from build123d import *

# Parameters (mm, degrees)
SKETCH1_R           = 8.89
SKETCH1_R_2         = 6.35
BOSS_EXTRUDE1_DEPTH = 13.462
SKETCH3_R           = 8.89
SKETCH3_R_2         = 6.35
SKETCH5_R           = 8.89
SKETCH5_R_2         = 6.349329507
BOSS_EXTRUDE2_DEPTH = 13.462


with BuildPart() as part:
    # Sketch1 → Boss-Extrude1 (new body)
    with BuildSketch(Plane(origin=(0, 0, 0), x_dir=(1, 0, 0), z_dir=(0, 1, 0))):
        with Locations(Location((0, 0, 0), (0, 0, 270))):
            Circle(SKETCH1_R)
        with Locations(Location((0, 0, 0), (0, 0, 270))):
            Circle(SKETCH1_R_2, mode=Mode.SUBTRACT)
    extrude(amount=BOSS_EXTRUDE1_DEPTH)

    # Sweep1: sweep along a path in Sketch2
    with BuildLine(Plane(origin=(0, 0, 0), x_dir=(0, 0, -1), z_dir=(1, 0, 0))) as sweep1_path:
        ThreePointArc((0, 0), (-3.719743879, -8.980256121), (-12.7, -12.7))
    # Sketch3 → Sweep1 (sweep)
    with BuildSketch(Plane.XZ):
        Circle(SKETCH3_R)
        Circle(SKETCH3_R_2, mode=Mode.SUBTRACT)
    sweep(path=sweep1_path.line)

    # Sketch5 → Boss-Extrude2 (add)
    with BuildSketch(Plane.XY.offset(12.7)):
        with Locations(Location((0, -12.7, 0), (0, 0, 270))):
            Circle(SKETCH5_R)
        with Locations(Location((0, -12.7, 0), (0, 0, 270))):
            Circle(SKETCH5_R_2, mode=Mode.SUBTRACT)
    extrude(amount=BOSS_EXTRUDE2_DEPTH)


solid = part.part
Geometry: final body of the model. Coordinates: model frame, mm. A direction names the side the tool comes from. Give positions to 0.01 mm unless a question says otherwise; leave off trailing zeros. Loops run counter-clockwise (first coordinate to the right, second up) from the corner with the lowest first, then second, coordinate; pieces in that order, holes last. Notation, with made-up numbers: (0.5, -6) - (16.5, -6) arc R10 ccw to (16.5, 12) - close; hole circle Ø2 at (10, 76). An arc over 180 degrees is marked (long way). One line per question, with ' | ' between items. Start each with the question number.
(1) Section query B-B on y = 4. Return loops of the section in (x, z).
(2) Ray query, line 1 (Y direction, x = 0, z = 23); line 2 (X direction, y = -12.7, z = 19.25); line 3 (Z direction, x = 2, y = 7). Return the intervals inside material, ascending. Write a range as from..to.
(3) Section query D-D on x = 7. Return loops of the section in (y, z).
(4) Reachability of faces 4 (the cylindrical face through (-8.68, 6.64, -1.93)), 5 (the flat face through (-6, 13.462, 4)), 6 (the cylindrical face through (-3.86, -7.66, 19.34)) from +Z, -Z, +X, -X, +Y, -Y: full face, straight path, thin tool, end or side. Return the list, or none.
(5) Contact query for flat-ended pins moving along their axis: pin 1 (1 mm diameter, centred on x = -2, y = -17, fed in from -Z); pin 2 (1.5 mm diameter, centred on x = -2.5, y = -12.5, fed in from -Z); pin 3 (2 mm diameter, centred on x = 0.5, y = -15, fed in from +Z). Output: stop coordinate, or through.
(6) Section query C-C on z = 22. Return loops of the section in (x, y), then the cut area to 3 significant figures.
(7) Pull-direction query (Z, two-part tool) for faces 1 (the cylindrical face through (-3.86, 6.64, -5.04)), 2 (the flat face through (-6, -17, 26.162)), 3 (the cylindrical face through (-5.409, -5.645, 19.337)); classes: released by +Z, released by -Z, zero draft, split by the parting line, or undercut.
The answers:
1) outline: circle Ø17.78 at (0, 0); hole circle Ø12.7 at (0, 0)
2) line 1: -21.59..-19.05, -6.35..-3.81 | line 2: -8.89..-6.35, 6.35..8.89 | line 3: -8.66..-6.03, 6.03..8.66
3) outline: (-18.18, 12.7) arc R18.18 ccw to (0, -5.48) - (13.46, -5.48) - (13.46, 5.48) - (0, 5.48) arc R7.22 cw to (-7.22, 12.7) - (-7.22, 26.16) - (-18.18, 26.16) - close
4) face 4: +Y | face 5: +Z, -Z, +X, -X, +Y | face 6: +Z
5) pin 1: z = -0.89 | pin 2: z = -5.04 | pin 3: z = 2.41
6) outline: circle Ø17.78 at (0, -12.7); hole circle Ø12.7 at (0, -12.7) | area: 122 mm2
7) face 1: undercut | face 2: released by +Z | face 3: zero draft
